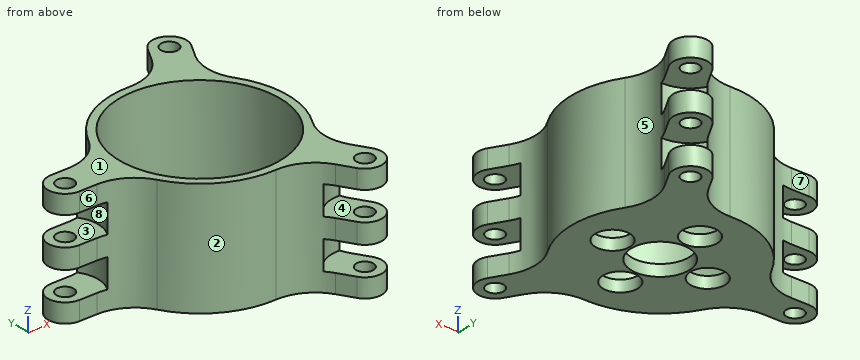
```python
from build123d import *

# Parameters (mm, degrees)
SKETCH1_R                 = 15.4
BOSS_EXTRUDE1_DEPTH       = 20
BOSS_EXTRUDE2_DEPTH       = 20
FILLET4_R                 = 8
CIRPATTERN11_COUNT        = 3
FILLET4_OF_CIRPATTERN11_R = 8
SKETCH4_R                 = 14
CUT_EXTRUDE3_DEPTH        = 18
SKETCH5_R                 = 5
CUT_EXTRUDE4_DEPTH        = 19
CUT_EXTRUDE4_DEPTH_BACK   = 3
CUT_EXTRUDE5_START        = -3
SKETCH7_R                 = 3
CUT_EXTRUDE5_DEPTH        = 22
CIRPATTERN12_COUNT        = 4
CUT_EXTRUDE1_START        = -21
SKETCH2_R                 = 1.5
CUT_EXTRUDE1_DEPTH        = 22
CIRPATTERN10_COUNT        = 3
SKETCH3_R                 = 5.75
CUT_EXTRUDE2_DEPTH        = 2.5
CIRPATTERN3_COUNT         = 3
MIRROR1_COPY_1_SKETCH_R   = 5.75
MIRROR1_COPY_1_DEPTH      = 2.5
MIRROR1_COPY_2_SKETCH_R   = 5.75
MIRROR1_COPY_2_DEPTH      = 2.5


with BuildPart() as part:
    # Sketch1 → Boss-Extrude1 (new body)
    with BuildSketch(Plane.XY):
        Circle(SKETCH1_R)
    extrude(amount=BOSS_EXTRUDE1_DEPTH)

    # Sketch6 → Boss-Extrude2 (add)
    with BuildSketch(Plane.XY.offset(20)):
        with BuildLine():
            Line((-23.775, 3), (-15.104966071, 3))
            ThreePointArc((-15.104966071, 3), (-15.4, 0), (-15.104966071, -3))
            Line((-15.104966071, -3), (-23.775, -3))
            ThreePointArc((-23.775, -3), (-26.775, 0), (-23.775, 3))
        make_face()
    boss_extrude2 = extrude(amount=-BOSS_EXTRUDE2_DEPTH)

    # Fillet4
    fillet4_edges = [part.edges().sort_by_distance(p)[0] for p in [
        (-15.104966071, 3, 10),
        (-15.104966071, -3, 10),
    ]]
    fillet(fillet4_edges, radius=FILLET4_R)

    # CirPattern11: Boss-Extrude2 ×3 about axis
    cirpattern11_axis = Axis((0, 0, 0), (0, 0, 1))
    for i in range(1, CIRPATTERN11_COUNT):
        add(boss_extrude2.rotate(cirpattern11_axis, i * 360 / CIRPATTERN11_COUNT))

    # Fillet4 of CirPattern11
    fillet4_of_cirpattern11_edges = [part.edges().sort_by_distance(p)[0] for p in [
        (4.954406824, -14.581284341, 10),
        (10.150559247, -11.581284341, 10),
        (10.150559247, 11.581284341, 10),
        (4.954406824, 14.581284341, 10),
    ]]
    fillet(fillet4_of_cirpattern11_edges, radius=FILLET4_OF_CIRPATTERN11_R)

    # Sketch4 → Cut-Extrude3 (cut)
    with BuildSketch(Plane.XY.offset(20)):
        Circle(SKETCH4_R)
    extrude(amount=-CUT_EXTRUDE3_DEPTH, mode=Mode.SUBTRACT)

    # Sketch5 → Cut-Extrude4 (cut, two sides)
    with BuildSketch(Plane.XY.offset(2)) as cut_extrude4_sk:
        Circle(SKETCH5_R)
    extrude(amount=CUT_EXTRUDE4_DEPTH, mode=Mode.SUBTRACT)
    extrude(cut_extrude4_sk.sketch, amount=-CUT_EXTRUDE4_DEPTH_BACK, mode=Mode.SUBTRACT)

    # Sketch7 → Cut-Extrude5 (cut)
    with BuildSketch(Plane.XY.offset(2).offset(CUT_EXTRUDE5_START)):
        with Locations((-8.4, 0)):
            Circle(SKETCH7_R)
    cut_extrude5 = extrude(amount=CUT_EXTRUDE5_DEPTH, mode=Mode.SUBTRACT)

    # CirPattern12: Cut-Extrude5 ×4 about axis
    cirpattern12_axis = Axis((0, 0, 0), (0, 0, 1))
    for i in range(1, CIRPATTERN12_COUNT):
        add(cut_extrude5.rotate(cirpattern12_axis, i * 360 / CIRPATTERN12_COUNT), mode=Mode.SUBTRACT)

    # Sketch2 → Cut-Extrude1 (cut)
    with BuildSketch(Plane.XY.offset(20).offset(CUT_EXTRUDE1_START)):
        with Locations((-23.775, 0)):
            Circle(SKETCH2_R)
    cut_extrude1 = extrude(amount=CUT_EXTRUDE1_DEPTH, mode=Mode.SUBTRACT)

    # CirPattern10: Cut-Extrude1 ×3 about axis
    cirpattern10_axis = Axis((0, 0, 0), (0, 0, 1))
    for i in range(1, CIRPATTERN10_COUNT):
        add(cut_extrude1.rotate(cirpattern10_axis, i * 360 / CIRPATTERN10_COUNT), mode=Mode.SUBTRACT)

    # Sketch3 → Cut-Extrude2 (cut, symmetric)
    with BuildSketch(Plane.XY.offset(5.771567898)):
        with Locations((-23.775, 0)):
            Circle(SKETCH3_R)
    cut_extrude2 = extrude(amount=CUT_EXTRUDE2_DEPTH, both=True, mode=Mode.SUBTRACT)

    # CirPattern3: Cut-Extrude2 ×3 about axis
    cirpattern3_axis = Axis((0, 0, 0), (0, 0, 1))
    for i in range(1, CIRPATTERN3_COUNT):
        add(cut_extrude2.rotate(cirpattern3_axis, i * 360 / CIRPATTERN3_COUNT), mode=Mode.SUBTRACT)

    # Mirror1: Cut-Extrude2 across plane
    add(cut_extrude2.mirror(Plane.XY.offset(10)), mode=Mode.SUBTRACT)

    # Mirror1 copy 1 sketch → Mirror1 copy 1 (cut, symmetric)
    with BuildSketch(Plane(origin=(0, 0, 14.228432102), x_dir=(-0.5, 0.866025404, 0), z_dir=(0, 0, -1))):
        with Locations((-23.775, 0)):
            Circle(MIRROR1_COPY_1_SKETCH_R)
    extrude(amount=MIRROR1_COPY_1_DEPTH, both=True, mode=Mode.SUBTRACT)

    # Mirror1 copy 2 sketch → Mirror1 copy 2 (cut, symmetric)
    with BuildSketch(Plane(origin=(0, 0, 14.228432102), x_dir=(-0.5, -0.866025404, 0), z_dir=(0, 0, -1))):
        with Locations((-23.775, 0)):
            Circle(MIRROR1_COPY_2_SKETCH_R)
    extrude(amount=MIRROR1_COPY_2_DEPTH, both=True, mode=Mode.SUBTRACT)


solid = part.part
```
CAD build for the part. Positions are in the model's coordinates, mm. Face numbers are marked on the shaded views. A direction names the side the tool comes from. Round coordinates to 2 decimals unless told otherwise and drop trailing zeros. Order: outer loops, then holes, each group sorted by start corner. A loop starts at its lowest first (then second) coordinate and runs counter-clockwise, first axis right, second up.
Item 1: Saw through at B-B on y = -4. Write the cut outline in (x, z).
Item 2: Pin check, flat tips, straight feed: pin 1 (2.5 mm diameter, centred on x = 11.89, y = 20.59, fed in from -Z); pin 2 (1.5 mm diameter, centred on x = -1.5, z = 7.5, fed in from +Y); pin 3 (4 mm diameter, centred on x = 10, y = 19, fed in from -Z); pin 4 (9.5 mm diameter, centred on x = 0, y = 8.4, fed in from +Z). Stop position of each tip, or through.
Item 3: Mould opens along Z. For the marked faces 1, 2 and 3 say: pulls with the +Z half, pulls with the -Z half, needs draft (parallel to the pull), parting line crosses it, or undercut.
Item 4: Tool access for the marked faces 4, 5, 6, 7 and 8: list every direction of +Z, -Z, +X, -X, +Y, -Y with a clear straight run to the whole face (end or side of a thin tool).
Item 5: Probe line 1 along Y through (x, z) = (0.5, 13.25); line 2 along Z through (x, y) = (-7.5, 11); line 3 along Y through (x, z) = (-10.5, 10). List the from-to ranges inside material, lowest first.
Item 6: Saw through at D-D on y = -20.5. Write the cut outline in (x, z), then the cut area to 3 significant figures.
Item 7: Saw through at A-A on x = -8.4. Write the cut outline in (y, z), then the cut area to 3 significant figures.
Reported:
1. outline: (-16.78, 0) - (-3, 0) - (-3, 2) - (-13.42, 2) - (-13.42, 20) - (-16.78, 20) - close; (3, 0) - (14.87, 0) - (14.87, 20) - (13.42, 20) - (13.42, 2) - (3, 2) - close
2. pin 1: passes through
2. pin 2: stops at y = 15.38
2. pin 3: stops at z = 0
2. pin 4: stops at z = 2
3. face 1: pulls with the +Z half
3. face 2: needs draft
3. face 3: undercut
4. face 4: +X, -Y
4. face 5: +Z, -Z, +X
4. face 6: +Z, -Z, -X, -Y
4. face 7: +Z, -Z, -X, +Y
4. face 8: -X
5. line 1: y = -15.39 to -13.99, 13.99 to 15.39
5. line 2: z = 0 to 2
5. line 3: y = -11.27 to -9.26, 9.26 to 11.27
6. outline: (8.37, 0) - (10.39, 0) - (10.39, 3.27) - (8.37, 3.27) - close; (8.37, 8.27) - (10.39, 8.27) - (10.39, 11.73) - (8.37, 11.73) - close; (8.37, 16.73) - (10.39, 16.73) - (10.39, 20) - (8.37, 20) - close; (13.38, 0) - (14.89, 0) - (14.89, 3.27) - (13.38, 3.27) - close; (13.38, 8.27) - (14.89, 8.27) - (14.89, 11.73) - (13.38, 11.73) - close; (13.38, 16.73) - (14.89, 16.73) - (14.89, 20) - (13.38, 20) - close
6. area: 35.2 mm2
7. outline: (-12.91, 0) - (-3, 0) - (-3, 2) - (-11.2, 2) - (-11.2, 20) - (-12.91, 20) - close; (3, 0) - (12.91, 0) - (12.91, 20) - (11.2, 20) - (11.2, 2) - (3, 2) - close
7. area: 101 mm2
